from build123d import *

# Parameters (mm, degrees)
BOSS_EXTRUDE1_DEPTH = 0.69
CUT_EXTRUDE1_DEPTH  = 1.69
SKETCH3_W           = 6
SKETCH3_H           = 28
CUT_EXTRUDE2_DEPTH  = 0.14
FILLET1_R           = 6


with BuildPart() as part:
    # Sketch1 → Boss-Extrude1 (new body)
    with BuildSketch(Plane(origin=(0, 0, 0), x_dir=(1, 0, 0), z_dir=(0, 1, 0))):
        Polygon((-146, 129), (-146, -43), (-129, -60), (-129, -129), (129, -129), (129, -36), (137, -28), (137, 28), (129, 36), (129, 129), align=None)
    extrude(amount=BOSS_EXTRUDE1_DEPTH)

    # Sketch2 → Cut-Extrude1 (cut, through all)
    with BuildSketch(Plane(origin=(0, 0.69, 0), x_dir=(1, 0, 0), z_dir=(0, 1, 0))):
        with BuildLine():
            Line((131, 20.875), (131, -20.875))
            ThreePointArc((131, -20.875), (130, -21.875), (129, -20.875))
            Line((129, -20.875), (129, 20.875))
            ThreePointArc((129, 20.875), (130, 21.875), (131, 20.875))
        make_face()
    extrude(amount=-CUT_EXTRUDE1_DEPTH, mode=Mode.SUBTRACT)

    # Sketch3 → Cut-Extrude2 (cut)
    with BuildSketch(Plane(origin=(0, 0.69, 0), x_dir=(1, 0, 0), z_dir=(0, 1, 0))):
        with Locations((134, 0)):
            Rectangle(SKETCH3_W, SKETCH3_H)
    extrude(amount=-CUT_EXTRUDE2_DEPTH, mode=Mode.SUBTRACT)

    # Fillet1
    fillet1_edges = [part.edges().sort_by_distance(p)[0] for p in [
        (129, 0.345, 36),
        (129, 0.345, 129),
        (-129, 0.345, 129),
        (-129, 0.345, 60),
        (-146, 0.345, 43),
        (-146, 0.345, -129),
        (129, 0.345, -129),
        (129, 0.345, -36),
        (137, 0.345, -28),
        (137, 0.345, 28),
    ]]
    fillet(fillet1_edges, radius=FILLET1_R)


solid = part.part
Geometry: final body of the model. Coordinates: model frame, mm. Give positions to 0.01 mm unless a question says otherwise; leave off trailing zeros. Loops run counter-clockwise (first coordinate to the right, second up) from the corner with the lowest first, then second, coordinate; pieces in that order, holes last. Notation, with made-up numbers: (29.5, -31) -> (56.5, -31) arc R10 cw to (56.5, -12) -> close; hole circle Ø4 at (-26, -2). An arc over 180 degrees is marked (long way). Put each result on its own line as item: value.
1. Cut plane A-A (y = 0.4). Return the cut outline in (x, z) (3 decimals).
Taken from the geometry:
outline: (-146, -123) arc R6 ccw to (-140, -129) -> (123, -129) arc R6 ccw to (129, -123) -> (129, -38.485) arc R6 cw to (130.757, -34.243) -> (135.243, -29.757) arc R6 ccw to (137, -25.515) -> (137, 25.515) arc R6 ccw to (135.243, 29.757) -> (130.757, 34.243) arc R6 cw to (129, 38.485) -> (129, 123) arc R6 ccw to (123, 129) -> (-123, 129) arc R6 ccw to (-129, 123) -> (-129, 62.485) arc R6 cw to (-130.757, 58.243) -> (-144.243, 44.757) arc R6 ccw to (-146, 40.515) -> close; hole (129, -20.875) arc R1 ccw to (131, -20.875) -> (131, 20.875) arc R1 ccw to (129, 20.875) -> close
2. Pull-direction query (Y, two-part tool) for faces 1 (the flat face through (134, 0.55, 0)), 2 (the flat face through (-6, 0, -2)), 3 (the cylindrical face through (127.196, 0.35, 127.289)); classes: released by +Y, released by -Y, zero draft, split by the parting line, or undercut.
Taken from the geometry:
face 1: released by +Y
face 2: released by -Y
face 3: zero draft
3. Ray query, line 1 along X through (y, z) = (0.1, -19); line 2 along X through (y, z) = (0.15, 84); line 3 along X through (y, z) = (0.6, 48.5). Return the intervals inside material, ascending. Write a range as [from, to].
Taken from the geometry:
line 1: x = [-146, 129], [131, 137]
line 2: x = [-129, 129]
line 3: x = [-140.5, 129]
4. Pin query (flat end, axial travel): P1, Ø1.8, axis at x = 135, z = 1.5, coming from the +Y side. Return the tip coordinate at first contact, or that it passes through.
Taken from the geometry:
P1: stops at y = 0.55
5. Cut plane B-B (z = -95). Return the cut outline in (x, y).
Taken from the geometry:
outline: (-146, 0) -> (129, 0) -> (129, 0.69) -> (-146, 0.69) -> close
